The listing builds one solid part. Answer for the finished solid, in the listing's coordinates (mm). Face numbers are marked on the shaded views. Give positions to 0.01 mm unless a question says otherwise; leave off trailing zeros. Order: outer loops, then holes, each group sorted by start corner. A loop starts at its lowest first (then second) coordinate and runs counter-clockwise, first axis right, second up. Notation, with made-up numbers: (46.25, 67.25) - (63.25, 67.25) arc R23 cw to (63.25, 90.25) - close; hole circle Ø2 at (65, 13.25). An arc over 180 degrees is marked (long way). Write each question's results on one line, items separated by ' | '. Start each with the question number.
1. Find the intervals of material crossed by L1, parallel to Z at x = 25, y = 8.25; L2, parallel to Y at x = -24, z = 0; L3, parallel to X at y = 23.5, z = -4, in increasing order.
2. Flat-ended cylindrical pins translate along their axes: pin 1 (2 mm diameter, centred on x = 23.5, y = 25.5, fed in from +Z); pin 2 (2 mm diameter, centred on x = -5, z = 4.5, fed in from +Y). Find the tip coordinate at first contact, or state that the pin passes through.
3. Section A-A (y = 4.5) is taken. Give the vertices of the cut face in (x, z).
4. Determine the mould class of the marked faces 1, 2, 3 and 4 for opening direction X: released by +X, released by -X, zero draft, split by the parting line, or undercut.
5. Section D-D (z = -1) is taken. Give the vertices of the cut face in (x, y), and give its area (3 significant figures).
6. Section C-C (x = -2) is taken. Give the vertices of the cut face in (y, z).
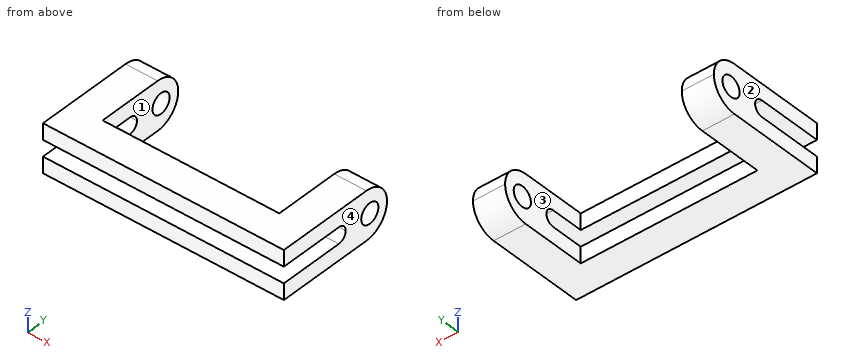
from build123d import *

# Parameters (mm, degrees)
SKETCH1_W           = 60
SKETCH1_H           = 12
BOSS_EXTRUDE1_DEPTH = 8
SKETCH2_W           = 8
SKETCH2_H           = 12
BOSS_EXTRUDE2_DEPTH = 22
SKETCH3_R           = 2.5
CUT_EXTRUDE1_DEPTH  = 68.349832962
FILLET1_R           = 6
SKETCH5_W           = 60
SKETCH5_H           = 4
CUT_EXTRUDE2_DEPTH  = 18
FILLET2_R           = 2


with BuildPart() as part:
    # Sketch1 → Boss-Extrude1 (new body)
    with BuildSketch(Plane(origin=(0, 0, 0), x_dir=(1, 0, 0), z_dir=(0, 1, 0))):
        Rectangle(SKETCH1_W, SKETCH1_H)
    extrude(amount=BOSS_EXTRUDE1_DEPTH)

    # Sketch2 → Boss-Extrude2 (add)
    with BuildSketch(Plane(origin=(0, 8, 0), x_dir=(1, 0, 0), z_dir=(0, 1, 0))):
        with Locations((-26, 0)):
            Rectangle(SKETCH2_W, SKETCH2_H)
        with Locations((26, 0)):
            Rectangle(SKETCH2_W, SKETCH2_H)
    extrude(amount=BOSS_EXTRUDE2_DEPTH)

    # Sketch3 → Cut-Extrude1 (cut, through all)
    with BuildSketch(Plane.ZY.offset(30)):
        with Locations((0, 25)):
            Circle(SKETCH3_R)
    extrude(amount=-CUT_EXTRUDE1_DEPTH, mode=Mode.SUBTRACT)

    # Fillet1
    fillet1_edges = [part.edges().sort_by_distance(p)[0] for p in [
        (-26, 30, 6),
        (26, 30, 6),
        (26, 30, -6),
        (-26, 30, -6),
    ]]
    fillet(fillet1_edges, radius=FILLET1_R - 0.0001)  # a hair under: the kernel refuses the full size

    # Sketch5 → Cut-Extrude2 (cut)
    with BuildSketch(Plane.XZ):
        Rectangle(SKETCH5_W, SKETCH5_H)
    extrude(amount=-CUT_EXTRUDE2_DEPTH, mode=Mode.SUBTRACT)

    # Fillet2
    fillet2_edges = [part.edges().sort_by_distance(p)[0] for p in [
        (-26, 18, 2),
        (-26, 18, -2),
        (26, 18, -2),
        (26, 18, 2),
    ]]
    fillet(fillet2_edges, radius=FILLET2_R - 0.0001)  # a hair under: the kernel refuses the full size


solid = part.part
Reported:
1) L1: -6 to -2, 2 to 6 | L2: 18 to 22.5, 27.5 to 30 | L3: -30 to -22, 22 to 30
2) pin 1: z = 5.98 | pin 2: y = 8
3) outline: (-30, -6) - (30, -6) - (30, -2) - (-30, -2) - close; (-30, 2) - (30, 2) - (30, 6) - (-30, 6) - close
4) face 1: undercut | face 2: released by -X | face 3: undercut | face 4: released by +X
5) outline: (-30, 17.73) - (-22, 17.73) - (-22, 22.71) - (-30, 22.71) - close; (-30, 27.29) - (-22, 27.29) - (-22, 29.92) - (-30, 29.92) - close; (22, 17.73) - (30, 17.73) - (30, 22.71) - (22, 22.71) - close; (22, 27.29) - (30, 27.29) - (30, 29.92) - (22, 29.92) - close | area: 122 mm²
6) outline: (0, -6) - (8, -6) - (8, -2) - (0, -2) - close; (0, 2) - (8, 2) - (8, 6) - (0, 6) - close
